from build123d import *

# Parameters (mm, degrees)
SKETCH1_R                          = 12.446
EXTRUDE1_DEPTH                     = 6.0071
CHAMFER1_SIZE                      = 1.524
SKETCH2_R                          = 11.5951
EXTRUDE2_DEPTH                     = 0.99076
SKETCH3_R                          = 1.5875
EXTRUDE3_DEPTH                     = 6.3754
F_5_16_0_3125_DIAMETER_HOLE2_D     = 5.1562
F_5_16_0_3125_DIAMETER_HOLE2_DEPTH = 0.381
M3X0_5_TAPPED_HOLE1_D              = 2.5
M3X0_5_TAPPED_HOLE1_DEPTH          = 5.3086
M3X0_5_TAPPED_HOLE1_TIP            = 0.751075774


with BuildPart() as part:
    # Sketch1 → Extrude1 (new body, symmetric)
    with BuildSketch(Plane(origin=(0, 0, 0), x_dir=(1, 0, 0), z_dir=(0, 1, 0))):
        Circle(SKETCH1_R)
    extrude(amount=EXTRUDE1_DEPTH, both=True)

    # Chamfer1
    chamfer1_edges = [part.edges().sort_by_distance(p)[0] for p in [
        (-12.446, 6.0071, 0),
    ]]
    chamfer(chamfer1_edges, length=CHAMFER1_SIZE)

    # Sketch2 → Extrude2 (add)
    with BuildSketch(Plane.XZ.offset(6.0071)):
        Circle(SKETCH2_R)
    extrude(amount=EXTRUDE2_DEPTH)

    # Sketch3 → Extrude3 (cut)
    with BuildSketch(Plane(origin=(0, 6.0071, 0), x_dir=(1, 0, 0), z_dir=(0, 1, 0))):
        Circle(SKETCH3_R)
    extrude(amount=-EXTRUDE3_DEPTH, mode=Mode.SUBTRACT)

    # Sketch4 → Cut-Revolve1 (revolve, cut)
    with BuildSketch(Plane.XY):
        with BuildLine():
            Line((0, 13.035099954), (0, -0.004899954))
            ThreePointArc((0, -0.004899954), (6.519999954, 6.5151), (0, 13.035099954))
        make_face()
    revolve(axis=Axis((0, 13.035099954, 0), (0, -1, 0)), mode=Mode.SUBTRACT)

    # 5/16 (0.3125) Diameter Hole2
    with Locations(Plane(origin=(12.446, 0, 0), x_dir=(0, 0, -1), z_dir=(1, 0, 0))):
        with Locations((0, -0.6223)):
            Hole(F_5_16_0_3125_DIAMETER_HOLE2_D / 2, depth=F_5_16_0_3125_DIAMETER_HOLE2_DEPTH)

    # M3x0.5 Tapped Hole1
    with Locations(Plane(origin=(12.065, 0, 0), x_dir=(0, 0, -1), z_dir=(1, 0, 0))):
        with Locations((0, -0.6223)):
            Hole(M3X0_5_TAPPED_HOLE1_D / 2, depth=M3X0_5_TAPPED_HOLE1_DEPTH)
            with Locations((0, 0, -(M3X0_5_TAPPED_HOLE1_DEPTH + M3X0_5_TAPPED_HOLE1_TIP / 2))):  # 118° drill point
                Cone(0, M3X0_5_TAPPED_HOLE1_D / 2, M3X0_5_TAPPED_HOLE1_TIP, mode=Mode.SUBTRACT)


solid = part.part
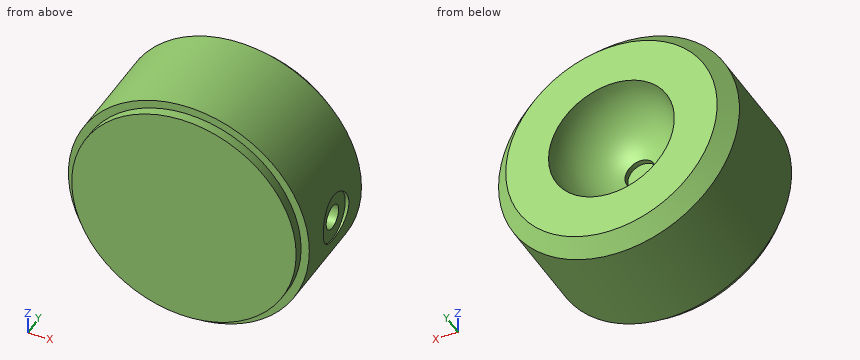
Work out the finished part from the listing and answer in its coordinate system (mm). Coordinates: 2 decimals unless noted, no trailing zeros. Write each loop counter-clockwise with the first axis right and the second up, starting at its lowest first coordinate (ties: lowest second). Pieces come first, ordered by that corner, then holes. Notation, with made-up numbers: M 56,88 L 78,88 A15 cw 78,106 Z; hole C -9.5,15.25 d1. An arc over 180 degrees is marked long. Use one line per item in the form item = value. Start each with the question number.
1. The part is cut by section A-A (x = 0). Give the vertices of the cut face in (y, z), plus the area to 3 significant figures.
2. Straight lines are drawn through the part: probe 1 along Z at (x, y) = (0, 0); probe 2 along X at (y, z) = (-0.1, 0); probe 3 along Y at (x, z) = (12.3, 0). For each, find the intervals that lie inside material, in ascending order. Write a range as from..to.
3. The part is cut by section B-B (y = 5.25). Give the vertices of the cut face in (x, z).
4. Each of these flat-tipped pins is pushed along its axis until it touches: P1, Ø3, axis at x = 2, z = -2, coming from the +Y side; P2, Ø1.5, axis at x = -7.5, y = 0.5, coming from the +Z side; P3, Ø4, axis at x = -4, y = 3.5, coming from the -Z side. Where does it stop, or does it pass through?
Evaluation:
q1.outline = M -7,-11.6 L -6.01,-11.6 L -6.01,-12.45 L 4.48,-12.45 L 6.01,-10.92 L 6.01,-6.5 A6.52 cw 0.19,-1.59 L -0.37,-1.59 L -0.37,1.59 L 0.19,1.59 A6.52 cw 6.01,6.5 L 6.01,10.92 L 4.48,12.45 L -6.01,12.45 L -6.01,11.6 L -7,11.6 Z
q1.area = 258 mm^2
q2.probe_1 = -12.45..-1.59, 1.59..12.45
q2.probe_2 = -12.45..-1.59, 1.59..6.32
q2.probe_3 = -6.01..-3.2, 1.96..4.63
q3.outline = C 0,0 d23.36; hole C 0,0 d12.79
q4.P1 = 1.64
q4.P2 = 10.46
q4.P3 = -12.28
